Verification items for the finished model (mm, model axes). Round coordinates to 2 decimals unless told otherwise and drop trailing zeros. Write each loop counter-clockwise with the first axis right and the second up, starting at its lowest first coordinate (ties: lowest second). Pieces come first, ordered by that corner, then holes. Notation, with made-up numbers: M -30,15.25 L -15,15.25 A28 ccw -15,38.25 Z; hole C 19,-12.5 d5. An arc over 180 degrees is marked long. Write each question's results on one line, items separated by ' | '.
from build123d import *

# Parameters (mm, degrees)
SKETCH1_W           = 150
SKETCH1_H           = 75
BOSS_EXTRUDE1_DEPTH = 5
CUT_EXTRUDE1_DEPTH  = 168.779617356
CUT_EXTRUDE2_DEPTH  = 168.779617356
SKETCH4_W           = 46
SKETCH4_H           = 45
CUT_EXTRUDE3_DEPTH  = 168.779617356
FILLET1_R           = 10
FILLET2_R           = 8


with BuildPart() as part:
    # Sketch1 → Boss-Extrude1 (new body)
    with BuildSketch(Plane(origin=(0, 0, 0), x_dir=(1, 0, 0), z_dir=(0, 1, 0))):
        with Locations((75, 37.5)):
            Rectangle(SKETCH1_W, SKETCH1_H)
    extrude(amount=BOSS_EXTRUDE1_DEPTH)

    # Sketch2 → Cut-Extrude1 (cut, through all)
    with BuildSketch(Plane(origin=(0, 5, 0), x_dir=(1, 0, 0), z_dir=(0, 1, 0))):
        with BuildLine():
            Line((13, 0), (13, 33))
            ThreePointArc((13, 33), (20, 40), (27, 33))
            Line((27, 33), (27, 0))
            Line((27, 0), (13, 0))
        make_face()
    extrude(amount=-CUT_EXTRUDE1_DEPTH, mode=Mode.SUBTRACT)

    # Sketch3 → Cut-Extrude2 (cut, through all)
    with BuildSketch(Plane(origin=(0, 5, 0), x_dir=(1, 0, 0), z_dir=(0, 1, 0))):
        with BuildLine():
            Line((137, 75), (137, 35))
            ThreePointArc((137, 35), (130, 28), (123, 35))
            Line((123, 35), (123, 75))
            Line((123, 75), (137, 75))
        make_face()
    extrude(amount=-CUT_EXTRUDE2_DEPTH, mode=Mode.SUBTRACT)

    # Sketch4 → Cut-Extrude3 (cut, through all)
    with BuildSketch(Plane(origin=(0, 5, 0), x_dir=(1, 0, 0), z_dir=(0, 1, 0))):
        with Locations((75, 37.5)):
            Rectangle(SKETCH4_W, SKETCH4_H)
    extrude(amount=-CUT_EXTRUDE3_DEPTH, mode=Mode.SUBTRACT)

    # Fillet1
    fillet1_edges = [part.edges().sort_by_distance(p)[0] for p in [
        (52, 2.5, -15),
        (52, 2.5, -60),
        (98, 2.5, -60),
        (98, 2.5, -15),
    ]]
    fillet(fillet1_edges, radius=FILLET1_R)

    # Fillet2
    fillet2_edges = [part.edges().sort_by_distance(p)[0] for p in [
        (0, 2.5, -75),
        (150, 2.5, -75),
        (150, 2.5, 0),
        (0, 2.5, 0),
    ]]
    fillet(fillet2_edges, radius=FILLET2_R)


solid = part.part
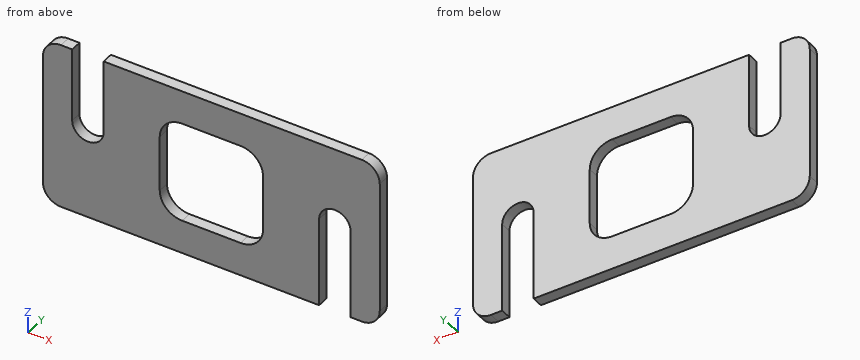
1) Material ranges on line 1 (X direction, y = 1.7, z = -48); line 2 (Z direction, x = 74, y = 2.6); line 3 (X direction, y = 2.6, z = -35), recorded low to high. Write a range as [from, to].
Calculated:
line 1: x = [0, 52], [98, 123], [137, 150] | line 2: z = [-75, -60], [-15, 0] | line 3: x = [0, 13.29], [26.71, 52], [98, 123], [137, 150]
2) Depth check by flat-ended pin: P1, Ø3, axis at x = 88.5, z = -12, coming from the -Y side. Enter the tip coordinate at first touch or a pass-through.
Calculated:
P1: stops at y = 0
3) Sectioned sample at A-A, the plane z = -58. Record the cut outline in (x, y), and give its area (3 significant figures).
Calculated:
outline: M 0,0 L 56,0 L 56,5 L 0,5 Z; M 94,0 L 123,0 L 123,5 L 94,5 Z; M 137,0 L 150,0 L 150,5 L 137,5 Z | area: 490 mm²
4) Sectioned sample at B-B, the plane y = 3.45. Record the cut outline in (x, z), and give its area (3 significant figures).
Calculated:
outline: M 0,-67 A8 ccw 8,-75 L 123,-75 L 123,-35 A7 cw 137,-35 L 137,-75 L 142,-75 A8 ccw 150,-67 L 150,-8 A8 ccw 142,0 L 27,0 L 27,-33 A7 cw 13,-33 L 13,0 L 8,0 A8 ccw 0,-8 Z; hole M 52,-50 A10 ccw 62,-60 L 88,-60 A10 ccw 98,-50 L 98,-25 A10 ccw 88,-15 L 62,-15 A10 ccw 52,-25 Z | area: 8,030 mm²
5) Sectioned sample at D-D, the plane x = 130. Record the cut outline in (y, z), and give its area (3 significant figures).
Calculated:
outline: M 0,-28 L 5,-28 L 5,0 L 0,0 Z | area: 140 mm²
6) Sectioned sample at C-C, the plane z = -30. Record the cut outline in (x, y).
Calculated:
outline: M 0,0 L 13,0 L 13,5 L 0,5 Z; M 27,0 L 52,0 L 52,5 L 27,5 Z; M 98,0 L 125.1,0 L 125.1,5 L 98,5 Z; M 134.9,0 L 150,0 L 150,5 L 134.9,5 Z
